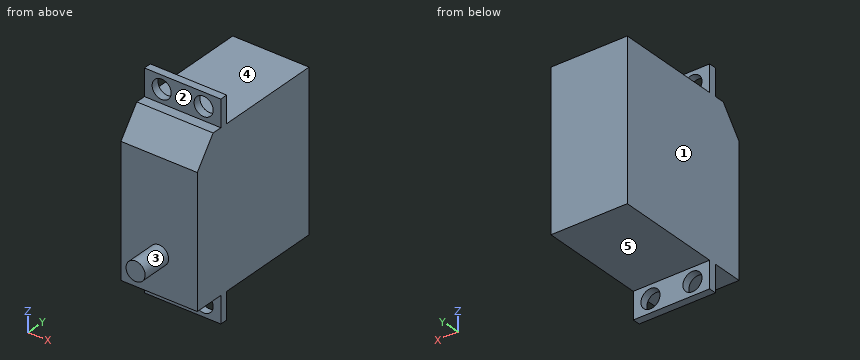
from build123d import *

# Parameters (mm, degrees)
SALIENTE_EXTRUIR1_DEPTH = 20
CROQUIS2_R              = 2.5
SALIENTE_EXTRUIR2_DEPTH = 8
CROQUIS3_R              = 2.5
CORTAR_EXTRUIR1_DEPTH   = 10


with BuildPart() as part:
    # Croquis1 → Saliente-Extruir1 (new body)
    with BuildSketch(Plane(origin=(0, 0, 0), x_dir=(0, 0, -1), z_dir=(1, 0, 0))):
        Polygon((41, 10), (48, 10), (48, 8), (41, 8), (41, 0), (7, 0), (0, 5.387789056), (0, 8), (-7, 8), (-7, 10), (0, 10), (0, 38), (41, 38), align=None)
    extrude(amount=SALIENTE_EXTRUIR1_DEPTH)

    # Croquis2 → Saliente-Extruir2 (add)
    with BuildSketch(Plane.XZ):
        with Locations(Location((10, -31, 0), (0, 0, 90))):
            Circle(CROQUIS2_R)
    extrude(amount=SALIENTE_EXTRUIR2_DEPTH)

    # Croquis3 → Cortar-Extruir1 (cut)
    with BuildSketch(Plane.XZ.offset(-8)):
        with Locations(Location((4.5, 3.5, 0), (0, 0, 270))):
            Circle(CROQUIS3_R)
        with Locations(Location((15.5, 3.5, 0), (0, 0, 270))):
            Circle(CROQUIS3_R)
        with Locations(Location((15.5, -44.5, 0), (0, 0, 270))):
            Circle(CROQUIS3_R)
        with Locations(Location((4.5, -44.5, 0), (0, 0, 270))):
            Circle(CROQUIS3_R)
    extrude(amount=-CORTAR_EXTRUIR1_DEPTH, mode=Mode.SUBTRACT)


solid = part.part
Verification items for the finished model (mm, model axes). Face numbers are marked on the shaded views. A direction names the side the tool comes from. Give positions to 0.01 mm unless a question says otherwise; leave off trailing zeros. Loops run counter-clockwise (first coordinate to the right, second up) from the corner with the lowest first, then second, coordinate; pieces in that order, holes last.
1) Set-up check for the marked faces 1, 2, 3, 4 and 5: record each of +Z, -Z, +X, -X, +Y, -Y from which the full face is reachable in a straight line by a thin tool's end or side.
2) Sectioned sample at C-C, the plane z = -23. Enter the section's corners in (x, y), then the cut area to 3 significant figures.
3) Sectioned sample at D-D, the plane y = 13. Enter the section's corners in (x, z).
4) Sectioned sample at B-B, the plane z = -44.5. Enter the section's corners in (x, y).
5) Thickness scan on line 1 along X through (y, z) = (8.9, 3.5); line 2 along X through (y, z) = (9, 2); line 3 along Z through (x, y) = (3.5, 5.5). Record the ranges inside material, lowest first.
6) Depth check by flat-ended pin: pin 1 Ø10 at (x, y) = (10.5, 18) entering from -Z; pin 2 Ø6 at (x, z) = (15.5, -44.5) entering from +Y; pin 3 Ø4 at (x, z) = (15.5, 3.5) entering from +Y; pin 4 Ø6 at (x, z) = (11.5, -23) entering from -Y. Enter the tip coordinate at first touch or a pass-through.
7) Sectioned sample at A-A, the plane x = 14. Enter the section's corners in (y, z), then the cut area to 3 significant figures.
Answers:
1. face 1: +Z, -Z, -X, +Y, -Y
1. face 2: +Z, +X, -X, -Y
1. face 3: -Y
1. face 4: +Z, +X, -X, +Y
1. face 5: -Z, +X, -X, +Y
2. outline: (0, 0) - (20, 0) - (20, 38) - (0, 38) - close
2. area: 760 mm2
3. outline: (0, -41) - (20, -41) - (20, 0) - (0, 0) - close
4. outline: (0, 8) - (2, 8) - (2, 10) - (0, 10) - close; (7, 8) - (13, 8) - (13, 10) - (7, 10) - close; (18, 8) - (20, 8) - (20, 10) - (18, 10) - close
5. line 1: x = 0 to 2, 7 to 13, 18 to 20
5. line 2: x = 0 to 2.5, 6.5 to 13.5, 17.5 to 20
5. line 3: z = -41 to 0
6. pin 1: stops at z = -41
6. pin 2: stops at y = 10
6. pin 3: passes through
6. pin 4: stops at y = 0
7. outline: (0, -41) - (8, -41) - (8, -42.5) - (10, -42.5) - (10, -41) - (38, -41) - (38, 0) - (10, 0) - (10, 1.5) - (8, 1.5) - (8, 0) - (5.39, 0) - (0, -7) - close; (8, -48) - (10, -48) - (10, -46.5) - (8, -46.5) - close; (8, 5.5) - (10, 5.5) - (10, 7) - (8, 7) - close
7. area: 1,550 mm2
